Verification items for the finished model (mm, model axes). A direction names the side the tool comes from. Coordinates: 2 decimals unless noted, no trailing zeros. Order: outer loops, then holes, each group sorted by start corner. A loop starts at its lowest first (then second) coordinate and runs counter-clockwise, first axis right, second up. Notation, with made-up numbers: M 0,-11 L 35,-11 A30 cw 35,14 Z; hole C 88,0 d2. An arc over 180 degrees is marked long. Answer as a JSON object with one key per item and string values. Group by question number.
(1) Material ranges on line 1 (X direction, y = 18.15, z = 0); line 2 (X direction, y = 6.75, z = 0); line 3 (Z direction, x = -2.5, y = 8), recorded low to high.
(2) Cross-section at C-C (y = 9.75). Count the separate pieces of the cut face and the enclosed holes in it, plus the area to 3 significant figures.
(3) Mould release check, pull along Z, two halves, no side actions. Record for faces 3 (the face through (8.631, 10.14, -19.106)), 4 (the face through (7.509, 9.86, 23.846)), 5 (the face through (-11, 20, 5)), 6 (the face through (10.676, 10.14, 19.467)): released by +Z, released by -Z, zero draft, split by the parting line, or undercut.
(4) Cross-section at A-A (x = 0). Enter the section's corners in (y, z).
(5) Gauge pin test, flat ends, axial feed: pin 1 Ø12 at (x, y) = (-16.5, 16.5) entering from -Z; pin 2 Ø8 at (x, y) = (6, 8.5) entering from -Z; pin 3 Ø2 at (x, z) = (2.5, 6.5) entering from +Y; pin 4 Ø2.5 at (x, z) = (10, -17.32) entering from -Y. Record the tip position at first contact, or that the pin passes through.
(6) Cross-section at D-D (x = 10). Enter the section's corners in (y, z), plus the area to 3 significant figures.
(7) Access from +Z, -Z, +X, -X, +Y, -Y to the whole of each face (thin tool, end or side, straight path). Record for faces 1 (the face through (3, 17, 5)), 2 (the face through (-17.77, 10.14, -0.29)).
(8) Cross-section at B-B (z = 0). Enter the section's corners in (x, y).
from build123d import *

# Parameters (mm, degrees)
SKETCH1_R           = 25
SKETCH1_R_2         = 5.5
BOSS_EXTRUDE1_DEPTH = 20
SKETCH2_R           = 11.25
CUT_EXTRUDE2_DEPTH  = 3
SKETCH3_R           = 2.25
CUT_EXTRUDE3_DEPTH  = 20
CIRPATTERN1_COUNT   = 3


with BuildPart() as part:
    # Sketch1 → Boss-Extrude1 (new body)
    with BuildSketch(Plane(origin=(0, 0, 0), x_dir=(1, 0, 0), z_dir=(0, 1, 0))):
        with Locations(Location((0, 0, 0), (0, 0, 270))):
            Circle(SKETCH1_R)
        with Locations(Location((0, 0, 0), (0, 0, 270))):
            Circle(SKETCH1_R_2, mode=Mode.SUBTRACT)
    extrude(amount=BOSS_EXTRUDE1_DEPTH)

    # Sketch2 → Cut-Extrude2 (cut)
    with BuildSketch(Plane(origin=(0, 20, 0), x_dir=(1, 0, 0), z_dir=(0, 1, 0))):
        with Locations(Location((0, 0, 0), (0, 0, 270))):
            Circle(SKETCH2_R)
    extrude(amount=-CUT_EXTRUDE2_DEPTH, mode=Mode.SUBTRACT)

    # Sketch3 → Cut-Extrude3 (cut)
    with BuildSketch(Plane(origin=(0, 20, 0), x_dir=(1, 0, 0), z_dir=(0, 1, 0))):
        with Locations(Location((10, -17.320508076, 0), (0, 0, 270))):
            Circle(SKETCH3_R)
    cut_extrude3 = extrude(amount=-CUT_EXTRUDE3_DEPTH, mode=Mode.SUBTRACT)

    # CirPattern1: Cut-Extrude3 ×3 about axis
    cirpattern1_axis = Axis((0, 0, 0), (0, 1, 0))
    for i in range(1, CIRPATTERN1_COUNT):
        add(cut_extrude3.rotate(cirpattern1_axis, i * 360 / CIRPATTERN1_COUNT), mode=Mode.SUBTRACT)


solid = part.part
Taken from the geometry:
{
 "1": {"line 1": "x = -25 to -22.25, -17.75 to -11.25, 11.25 to 25", "line 2": "x = -25 to -22.25, -17.75 to -5.5, 5.5 to 25", "line 3": "z = -24.87 to -4.9, 4.9 to 24.87"},
 "2": {"separate pieces": "1", "enclosed holes": "4", "area": "1,820 mm²"},
 "3": {"face 3": "undercut", "face 4": "split by the parting line", "face 5": "zero draft", "face 6": "undercut"},
 "4": {"outline": "M 0,-25 L 20,-25 L 20,-11.25 L 17,-11.25 L 17,-5.5 L 0,-5.5 Z; M 0,5.5 L 17,5.5 L 17,11.25 L 20,11.25 L 20,25 L 0,25 Z"},
 "5": {"pin 1": "stops at z = -22.69", "pin 2": "stops at z = -24.92", "pin 3": "stops at y = 17", "pin 4": "passes through"},
 "6": {"outline": "M 0,-22.91 L 20,-22.91 L 20,-19.57 L 0,-19.57 Z; M 0,-15.07 L 20,-15.07 L 20,-5.15 L 17,-5.15 L 17,5.15 L 20,5.15 L 20,15.07 L 0,15.07 Z; M 0,19.57 L 20,19.57 L 20,22.91 L 0,22.91 Z", "area": "706 mm²"},
 "7": {"face 1": "+Y", "face 2": "+Y, -Y"},
 "8": {"outline": "M -25,0 L -22.25,0 L -22.25,20 L -25,20 Z; M -17.75,0 L -5.5,0 L -5.5,17 L -11.25,17 L -11.25,20 L -17.75,20 Z; M 5.5,0 L 25,0 L 25,20 L 11.25,20 L 11.25,17 L 5.5,17 Z"}
}
